from build123d import *

# Parameters (mm, degrees)
F1_DEPTH = 31.75
F3_DEPTH = 25.4
F4_R     = 6.35
F5_DEPTH = 25.4
F6_W     = 12.7
F6_H     = 19.05
F7_DEPTH = 44.45
F9_DEPTH = 44.451


with BuildPart() as f1:
    # F0 (on Front) → F1 (new body)
    with BuildSketch(Plane.XZ):
        Polygon((6.35, 6.35), (6.35, 0), (44.45, 0), (44.45, 12.7), (57.15, 12.7), (57.15, 19.05), (44.45, 19.05), (44.45, 31.75), (0, 31.75), (0, 6.35), align=None)
    extrude(amount=F1_DEPTH)

    # F2 (on face) → F3 (join)
    with BuildSketch(Plane(origin=(0, 0, 0), x_dir=(-1, 0, 0), z_dir=(0, 1, 0))):
        Polygon((-107.95, 0), (-44.45, 0), (-44.45, 12.7), (-57.15, 12.7), (-57.15, 19.05), (-44.45, 19.05), (-44.45, 31.75), (0, 31.75), (0, 63.5), (-50.8, 63.5), (-107.95, 19.05), align=None)
        Polygon((-44.45, 0), (-6.35, 0), (-6.35, 6.35), (0, 6.35), (0, 31.75), (-44.45, 31.75), (-44.45, 19.05), (-57.15, 19.05), (-57.15, 12.7), (-44.45, 12.7), align=None)
    extrude(amount=F3_DEPTH)

    # F4 (on face) → F5 (cut, through all)
    with BuildSketch(Plane.XZ):
        with Locations((12.7, 50.8)):
            Circle(F4_R)
    extrude(amount=-F5_DEPTH, mode=Mode.SUBTRACT)

    # F6 (on face) → F7 (cut)
    with BuildSketch(Plane.YZ.offset(107.95)):
        with Locations((19.05, 9.525)):
            Rectangle(F6_W, F6_H)
    extrude(amount=-F7_DEPTH, mode=Mode.SUBTRACT)

    # F8 (on face) → F9 (cut, through all)
    with BuildSketch(Plane(origin=(0, 0, 19.05), x_dir=(1, 0, 0), z_dir=(0, 0, -1))):
        Polygon((107.95, -25.4), (107.95, -12.7), (85.725, -25.4), align=None)
    extrude(amount=-F9_DEPTH, mode=Mode.SUBTRACT)


solid = f1.part
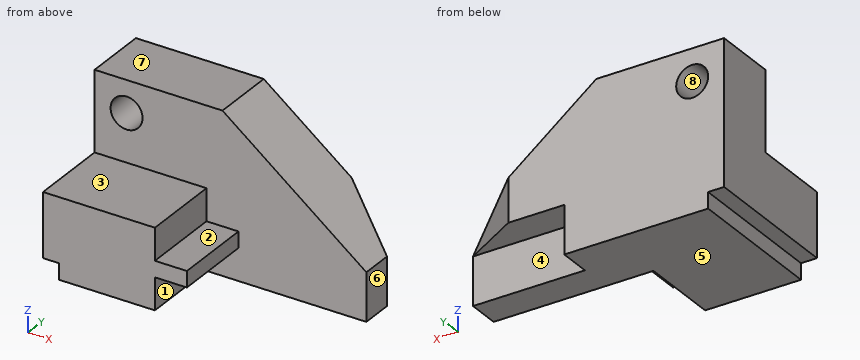
Verification items for the finished model (mm, model axes). Face numbers are marked on the shaded views. A direction names the side the tool comes from. Give positions to 0.01 mm unless a question says otherwise; leave off trailing zeros. Loops run counter-clockwise (first coordinate to the right, second up) from the corner with the lowest first, then second, coordinate; pieces in that order, holes last. Notation, with made-up numbers: (36, -11.5) - (95, -11.5) arc R18 cw to (95, 13.5) - close; hole circle Ø11 at (24.5, -36.75). An arc over 180 degrees is marked (long way). Write item = value, one per line. Start each with the question number.
Q1. Cross-section at C-C, the plane z = 50.8. Enter the section's corners in (x, y).
Q2. Tool access check on the marked faces 1, 2, 3, 4 and 5. Record the directions out of +Z, -Z, +X, -X, +Y, -Y that give a thin tool (end or side, any length) a straight path to the whole face; none if there is none.
Q3. Cross-section at B-B, the plane y = 7. Enter the section's corners in (x, z).
Q4. Cross-section at D-D, the plane y = -15. Enter the section's corners in (x, z).
Q5. Cross-section at A-A, the plane x = 12.7. Enter the section's corners in (y, z).
Q6. Depth check by flat-ended pin: P1, Ø7, axis at y = 3.5, z = 2.5, coming from the -X side; P2, Ø6.5, axis at y = -12, z = 28.5, coming from the +X side; P3, Ø6.5, axis at y = 18, z = 7.5, coming from the +X side. Enter the tip coordinate at first touch or a pass-through.
Q7. Thickness scan on line 1 (Z direction, x = 25, y = -23.5); line 2 (Z direction, x = 12, y = 15); line 3 (X direction, y = 18, z = 50). Record the ranges inside material, lowest first.
Q8. Mould release check, pull along X, two halves, no side actions. Record for the marked faces 6, 7 and 8: released by +X, released by -X, zero draft, split by the parting line, or undercut.
Answer key:
q1.outline = (0, 0) - (6.35, 0) - (6.35, 25.4) - (0, 25.4) - close; (19.05, 0) - (67.13, 0) - (67.13, 25.4) - (19.05, 25.4) - close
q2.face_1 = -Z, +X, -Y
q2.face_2 = +Z, +X, -Y
q2.face_3 = +Z, +X, -X, -Y
q2.face_4 = -Z, +X, +Y
q2.face_5 = -Z, +X, -X, +Y, -Y
q3.outline = (0, 6.35) - (6.35, 6.35) - (6.35, 0) - (107.95, 0) - (107.95, 19.05) - (50.8, 63.5) - (0, 63.5) - close; hole circle Ø12.7 at (12.7, 50.8)
q4.outline = (0, 6.35) - (6.35, 6.35) - (6.35, 0) - (44.45, 0) - (44.45, 12.7) - (57.15, 12.7) - (57.15, 19.05) - (44.45, 19.05) - (44.45, 31.75) - (0, 31.75) - close
q5.outline = (-31.75, 0) - (25.4, 0) - (25.4, 44.45) - (0, 44.45) - (0, 31.75) - (-31.75, 31.75) - close; (0, 57.15) - (25.4, 57.15) - (25.4, 63.5) - (0, 63.5) - close
q6.P1 = 6.35
q6.P2 = 44.45
q6.P3 = 63.5
q7.line_1 = 0 to 31.75
q7.line_2 = 0 to 44.49, 57.11 to 63.5
q7.line_3 = 0 to 6.4, 19 to 68.16
q8.face_6 = released by +X
q8.face_7 = zero draft
q8.face_8 = undercut
